Autodesk Inventor part; units mm, degrees
ref_plane "YZ Plane" through (0, 0, 0) normal (1, 0, 0) x (0, 1, 0)
ref_plane "XZ Plane" through (0, 0, 0) normal (0, 1, 0) x (-1, 0, 0)
ref_plane "XY Plane" through (0, 0, 0) normal (0, 0, 1) x (1, 0, 0)
sketch "Sketch1" plane through (0, 0, 0) normal (1, 0, 0) x (0, 1, 0)
  line L0 (27.65, 6.65) -> (-27.65, 6.65)
  line L1 (-27.65, 6.65) -> (-27.65, -6.65)
  line L2 (-27.65, -6.65) -> (27.65, -6.65)
  line L3 (27.65, -6.65) -> (27.65, 6.65)
  line L4 (27.65, 6.65) -> (-27.65, -6.65) construction
  line L5 (-27.65, 6.65) -> (27.65, -6.65) construction
  line L6 (30.65, -9.65) -> (-30.65, -9.65)
  line L7 (-30.65, -9.65) -> (-30.65, 9.65)
  line L8 (-30.65, 9.65) -> (30.65, 9.65)
  line L9 (30.65, 9.65) -> (30.65, -9.65)
  point P0 (0, 0)
  dimension "d0" = 55.3
  dimension "d1" = 13.3
  dimension "d2" = 3
extrude "Extrusion1" add sketch "Sketch1" along normal blind 12
sketch "Sketch2" plane through (12, 0, 0) normal (1, 0, 0) x (0, 0, -1)
  line L0 (-9.65, 30.65) -> (-9.65, -30.65)
  line L1 (-9.65, -30.65) -> (9.65, -30.65)
  line L2 (9.65, -30.65) -> (9.65, 30.65)
  line L3 (9.65, 30.65) -> (-9.65, 30.65)
  line L4 (-6.65, 27.65) -> (6.65, 27.65)
  line L5 (6.65, 27.65) -> (6.65, -27.65)
  line L6 (6.65, -27.65) -> (-6.65, -27.65)
  line L7 (-6.65, -27.65) -> (-6.65, 27.65)
  point P0 (0, 0)
extrude "Extrusion2" add sketch "Sketch2" against normal blind 11.5 contours L3 L2 L1 L0 | L4 L5 L6 L7
sketch "Sketch3" plane through (12, 0, 0) normal (1, 0, 0) x (0, 0, -1)
  line L0 (0, 0) -> (0, 21)
  line L1 (0, 0) -> (5, 0)
  circle A0 centre (0, 21) radius 2.65
  circle A1 centre (0, -21) radius 2.65
  dimension "d7" = 21
  dimension "d8" = 5
  dimension "d9" = 5.3
extrude "Extrusion3" cut sketch "Sketch3" against normal blind 13
fillet "Fillet1" radius 5 4 edges at (6, 30.65, 9.65) (6, 30.65, -9.65) (6, -30.65, -9.65) (6, -30.65, 9.65)
properties part number "TOPE_CHUMACERA"
Could you check a few things on this model? Use its own coordinates, in mm. A direction names the side the tool comes from. Round coordinates to 2 decimals unless told otherwise and drop trailing zeros. Write each loop counter-clockwise with the first axis right and the second up, starting at its lowest first coordinate (ties: lowest second). Pieces come first, ordered by that corner, then holes.
(1) For pin 1 (4 mm diameter, centred on y = 21, z = 0, fed in from -X); pin 2 (1 mm diameter, centred on y = -13.5, z = 3, fed in from -X), each with a flat end and sliding along its axis, tell me the tip position at first contact or that it passes through.
Findings below:
pin 1: passes through
pin 2: stops at x = 0.5
(2) Suppose I cut it at D-D on y = -2. Write out the boundary of the cut face in (x, z).
Findings below:
outline: (0, -9.65) - (12, -9.65) - (12, 9.65) - (0, 9.65) - (0, 6.65) - (0.5, 6.65) - (0.5, -6.65) - (0, -6.65) - close
(3) Suppose I cut it at C-C on x = 1.5. Write out the boundary of the cut face in (y, z), and give its area (3 significant figures).
Findings below:
outline: (-30.65, -4.65) arc R5 ccw to (-25.65, -9.65) - (25.65, -9.65) arc R5 ccw to (30.65, -4.65) - (30.65, 4.65) arc R5 ccw to (25.65, 9.65) - (-25.65, 9.65) arc R5 ccw to (-30.65, 4.65) - close; hole circle Ø5.3 at (-21, 0); hole circle Ø5.3 at (21, 0)
area: 1,120 mm2
(4) If I drill on probe 1 along Y at (x, z) = (6.75, 0); probe 2 along Z at (x, y) = (3.25, 21); probe 3 along X at (y, z) = (10, 4.5), over which ranges is the centre line in solid material (lowest first)?
Findings below:
probe 1: y = -30.65 to -23.65, -18.35 to 18.35, 23.65 to 30.65
probe 2: z = -9.65 to -2.65, 2.65 to 9.65
probe 3: x = 0.5 to 12
(5) Suppose I cut it at A-A on y = -21. Write out the boundary of the cut face in (x, z).
Findings below:
outline: (0, -9.65) - (12, -9.65) - (12, -2.65) - (0.5, -2.65) - (0.5, -6.65) - (0, -6.65) - close; (0, 6.65) - (0.5, 6.65) - (0.5, 2.65) - (12, 2.65) - (12, 9.65) - (0, 9.65) - close
(6) Which directions (+Z, -Z, +X, -X, +Y, -Y) give clear straight access to the entire face, cutting with the end or side of a thin tool? Please do faces 1 (the face through (0.5, 0, 0)), 2 (the face through (5.92, -29.15, -8.22)).
Findings below:
face 1: -X
face 2: -Z, +X, -X, -Y
(7) Suppose I cut it at B-B on z = 0. Write out the boundary of the cut face in (x, y), and give its area (3 significant figures).
Findings below:
outline: (0, -30.65) - (12, -30.65) - (12, -23.65) - (0.5, -23.65) - (0.5, -27.65) - (0, -27.65) - close; (0, 27.65) - (0.5, 27.65) - (0.5, 23.65) - (12, 23.65) - (12, 30.65) - (0, 30.65) - close; (0.5, -18.35) - (12, -18.35) - (12, 18.35) - (0.5, 18.35) - close
area: 586 mm2
(8) Thinking about a two-plate mould opening in Y: for faces 3 (the face through (6, 30.65, 0)), 4 (the face through (6, -30.65, 0)), 5 (the face through (6.33, -18.766, -1.425)), which applies, +Y half, -Y half, draft (parallel to the pull), parting line (faces both ways), or undercut?
Findings below:
face 3: +Y half
face 4: -Y half
face 5: undercut
